```python
from build123d import *

# Parameters (mm, degrees)
F0_W     = 114.3
F0_H     = 38.1
F1_DEPTH = 50.8
F2_DEPTH = 12.7
F3_R     = 5.08
F4_DEPTH = 55.88
F5_R     = 5.08


with BuildPart() as f1:
    # F0 (on Front) → F1 (new body)
    with BuildSketch(Plane.XZ):
        Polygon((63.5, -25.4), (63.5, 25.4), (57.15, 25.4), (0, 25.4), (-57.15, 25.4), (-63.5, 25.4), (-63.5, -25.4), align=None)
        Rectangle(F0_W, F0_H, mode=Mode.SUBTRACT)
    extrude(amount=F1_DEPTH)

    # F0 (on Front) → F2 (join)
    with BuildSketch(Plane.XZ):
        Rectangle(F0_W, F0_H)
    extrude(amount=F2_DEPTH)

    # F3
    f3_edges = [f1.edges().sort_by_distance(p)[0] for p in [
        (-63.5, -25.4, 25.4),
        (-63.5, -25.4, -25.4),
        (63.5, -25.4, -25.4),
        (63.5, -25.4, 25.4),
        (0, -50.8, 25.4),
        (-63.5, -50.8, 0),
        (0, -50.8, -25.4),
        (63.5, -50.8, 0),
    ]]
    fillet(f3_edges, radius=F3_R)

    # F0 (on Front) → F4 (join)
    with BuildSketch(Plane.XZ):
        Polygon((0, 25.4), (57.15, 25.4), (57.15, 63.5), (-57.15, 63.5), (-57.15, 25.4), align=None)
    extrude(amount=F4_DEPTH)

    # F5
    f5_edges = [f1.edges().sort_by_distance(p)[0] for p in [
        (-57.15, -27.94, 63.5),
        (57.15, -27.94, 63.5),
        (0, 0, 63.5),
    ]]
    fillet(f5_edges, radius=F5_R)


solid = f1.part
```
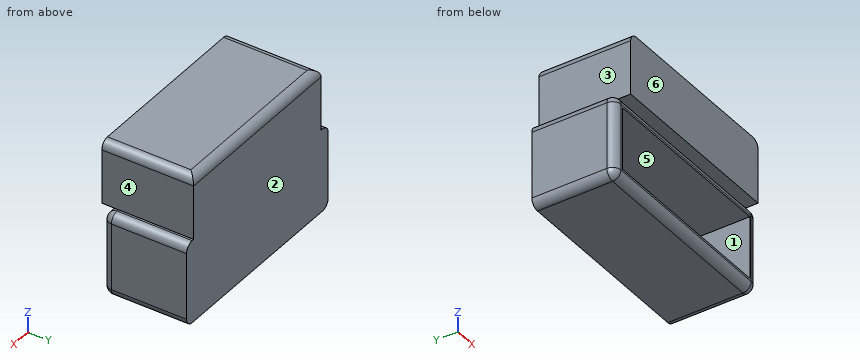
Verification items for the finished model (mm, model axes). Face numbers are marked on the shaded views. A direction names the side the tool comes from. Round coordinates to 2 decimals unless told otherwise and drop trailing zeros. Order: outer loops, then holes, each group sorted by start corner. A loop starts at its lowest first (then second) coordinate and runs counter-clockwise, first axis right, second up.
1) Tool access check on the marked faces 1, 2 and 3. Record the directions out of +Z, -Z, +X, -X, +Y, -Y that give a thin tool (end or side, any length) a straight path to the whole face; none if there is none.
Geometry says:
face 1: -Y
face 2: +Z, -Z, +X, -X, +Y
face 3: +Z, -X, +Y, -Y
2) Cross-section at B-B, the plane z = -11. Record the cut outline in (x, y), plus the area to 3 significant figures.
Geometry says:
outline: (-63.5, -45.72) arc R5.08 ccw to (-58.42, -50.8) - (-57.15, -50.8) - (-57.15, -12.7) - (57.15, -12.7) - (57.15, -50.8) - (58.42, -50.8) arc R5.08 ccw to (63.5, -45.72) - (63.5, 0) - (-63.5, 0) - close
area: 2,090 mm2
3) Cross-section at C-C, the plane x = 45.5. Record the cut outline in (y, z).
Geometry says:
outline: (-55.88, 25.4) - (-45.72, 25.4) arc R5.08 ccw to (-50.8, 20.32) - (-50.8, 19.05) - (-12.7, 19.05) - (-12.7, -19.05) - (-50.8, -19.05) - (-50.8, -20.32) arc R5.08 ccw to (-45.72, -25.4) - (0, -25.4) - (0, 58.42) arc R5.08 ccw to (-5.08, 63.5) - (-55.88, 63.5) - close
4) Depth check by flat-ended pin: pin 1 (1.5 mm diameter, centred on y = -12, z = 45, fed in from +X); pin 2 (16.5 mm diameter, centred on y = -24.5, z = 45, fed in from -X); pin 3 (4 mm diameter, centred on x = 49, z = 50, fed in from +Y); pin 4 (20.5 mm diameter, centred on x = -0.5, z = 3, fed in from -Y). Enter the tip coordinate at first touch or a pass-through.
Geometry says:
pin 1: stops at x = 57.15
pin 2: stops at x = -57.15
pin 3: stops at y = 0
pin 4: stops at y = -12.7
5) Material ranges on line 1 (X direction, y = -13.5, z = 5.5); line 2 (Z direction, x = -25, y = -32.5); line 3 (Y direction, x = -34.5, z = -12), recorded low to high.
Geometry says:
line 1: x = -63.5 to -57.15, 57.15 to 63.5
line 2: z = -25.4 to -19.05, 19.05 to 63.5
line 3: y = -12.7 to 0
6) Cross-section at A-A, the plane y = -48.5. Record the cut outline in (x, z).
Geometry says:
outline: (-62.67, -20.32) arc R4.25 ccw to (-58.42, -24.57) - (58.42, -24.57) arc R4.25 ccw to (62.67, -20.32) - (62.67, 20.32) arc R4.25 ccw to (58.42, 24.57) - (-58.42, 24.57) arc R4.25 ccw to (-62.67, 20.32) - close; (-57.15, 25.4) - (57.15, 25.4) - (57.15, 58.42) arc R5.08 ccw to (52.07, 63.5) - (-52.07, 63.5) arc R5.08 ccw to (-57.15, 58.42) - close; hole (-57.15, -19.05) - (57.15, -19.05) - (57.15, 19.05) - (-57.15, 19.05) - close
7) Cross-section at D-D, the plane y = -36.5. Record the cut outline in (x, z), plus the area to 3 significant figures.
Geometry says:
outline: (-63.5, -20.32) arc R5.08 ccw to (-58.42, -25.4) - (58.42, -25.4) arc R5.08 ccw to (63.5, -20.32) - (63.5, 20.32) arc R5.08 ccw to (58.42, 25.4) - (57.15, 25.4) - (57.15, 58.42) arc R5.08 ccw to (52.07, 63.5) - (-52.07, 63.5) arc R5.08 ccw to (-57.15, 58.42) - (-57.15, 25.4) - (-58.42, 25.4) arc R5.08 ccw to (-63.5, 20.32) - close; hole (-57.15, -19.05) - (57.15, -19.05) - (57.15, 19.05) - (-57.15, 19.05) - close
area: 6,420 mm2
8) Draft check along X on the marked faces 4, 5 and 6. Enter one of: +X half, -X half, draft (parallel to the pull), parting line (faces both ways), or undercut.
Geometry says:
face 4: +X half
face 5: undercut
face 6: draft
